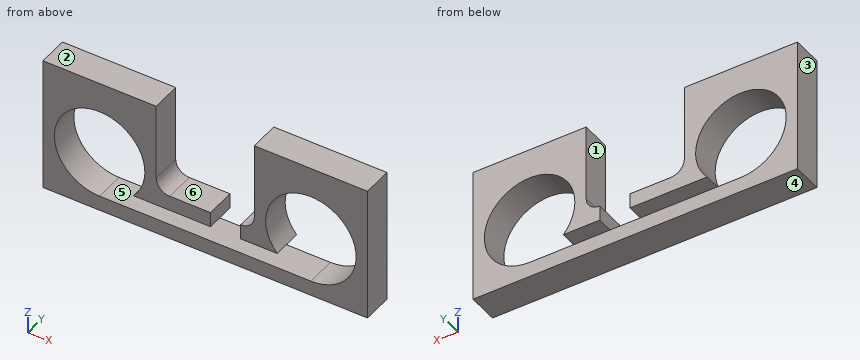
```python
from build123d import *

# Parameters (mm, degrees)
F0_W     = 273.05
F0_H     = 114.3
F1_DEPTH = 25.4
F2_R     = 38.1
F3_DEPTH = 25.4
F5_DEPTH = 25.4
F7_DEPTH = 25.4


with BuildPart() as f1:
    # F0 (on Front) → F1 (new body)
    with BuildSketch(Plane.XZ):
        with Locations((136.525, 57.15)):
            Rectangle(F0_W, F0_H)
    extrude(amount=F1_DEPTH)

    # F2 (on face) → F3 (cut)
    with BuildSketch(Plane.XZ.offset(25.4)):
        with Locations((47.625, 50.8)):
            Circle(F2_R)
        with Locations((225.425, 50.8)):
            Circle(F2_R)
    extrude(amount=-F3_DEPTH, mode=Mode.SUBTRACT)

    # F4 (on face) → F5 (cut)
    with BuildSketch(Plane.XZ.offset(25.4)):
        with BuildLine():
            Line((177.8, 114.3), (95.25, 114.3))
            Line((95.25, 114.3), (95.25, 49.53))
            ThreePointArc((95.25, 49.53), (98.597769, 41.447769), (106.68, 38.1))
            Line((106.68, 38.1), (166.37, 38.1))
            ThreePointArc((166.37, 38.1), (174.452231, 41.447769), (177.8, 49.53))
            Line((177.8, 49.53), (177.8, 114.3))
        make_face()
    extrude(amount=-F5_DEPTH, mode=Mode.SUBTRACT)

    # F6 (on face) → F7 (cut)
    with BuildSketch(Plane.XZ.offset(25.4)):
        Polygon((166.37, 25.4), (166.37, 38.1), (140.97, 38.1), (140.97, 25.4), (76.023063, 25.4), (47.625, 12.7), (166.37, 12.7), align=None)
        Polygon((197.026937, 25.4), (166.37, 25.4), (166.37, 12.7), (225.425, 12.7), align=None)
    extrude(amount=-F7_DEPTH, mode=Mode.SUBTRACT)


solid = f1.part
```
Can you work these out from the model? Positions are in its coordinate system, mm. Face numbers are marked on the shaded views. A direction names the side the tool comes from. Give positions to 0.01 mm unless a question says otherwise; leave off trailing zeros. Order: outer loops, then holes, each group sorted by start corner. A loop starts at its lowest first (then second) coordinate and runs counter-clockwise, first axis right, second up. Notation, with made-up numbers: (77.5, -18) - (130.5, -18) arc R17 cw to (130.5, -3) - close; hole circle Ø2 at (47.5, 7.5). An arc over 180 degrees is marked (long way). Use a Markdown table: item, result. Add a question column.
Q1. If we section it at A-A on z = 106: Write out the boundary of the cut face in (x, y).
Q2. If we mould it in two halves opening along X, with no side actions, what happens to the marked faces 1, 2 and 3? For each: released by +X, released by -X, zero draft, split by the parting line, or undercut.
Q3. If we section it at B-B on x = 243.5: Write out the boundary of the cut face in (y, z).
Q4. If we section it at D-D on y = -19: Write out the boundary of the cut face in (x, z) (3 decimals).
Q5. I'm going to push flat-ended pins straight in: pin 1 (12.5 mm diameter, centred on y = -6.5, z = 94, fed in from -X); pin 2 (7.5 mm diameter, centred on x = 124, y = -12.5, fed in from +Z); pin 3 (2 mm diameter, centred on x = 157, y = -17, fed in from +Z); pin 4 (2 mm diameter, centred on x = 244, z = 20.5, fed in from +Y). Where does each tip first touch, or does it pass through?
Q6. On a 3-axis mill with a long thin cutter (end or side, diameter ignored), from which of +Z, -Z, +X, -X, +Y, -Y can I reach the whole of each face in a straight line? I mean the marked faces 4, 5 and 6. Say none if no direction works.
Q7. If we section it at C-C on z = 58.5: Write out the boundary of the cut face in (x, y), plus the area to 3 significant figures.
Q8. Please list where these lines run through material, in increasing order: line 1 along X through (y, z) = (-11.75, 50.8) (3 decimals); line 2 along X through (y, z) = (-24.5, 100); line 3 along X through (y, z) = (-15.25, 86).
Answers follow:
| question | item | result |
|---|---|---|
| 1 | outline | (0, -25.4) - (95.25, -25.4) - (95.25, 0) - (0, 0) - close; (177.8, -25.4) - (273.05, -25.4) - (273.05, 0) - (177.8, 0) - close |
| 2 | face 1 | undercut |
| 2 | face 2 | zero draft |
| 2 | face 3 | released by -X |
| 3 | outline | (-25.4, 0) - (0, 0) - (0, 17.26) - (-25.4, 17.26) - close; (-25.4, 84.34) - (0, 84.34) - (0, 114.3) - (-25.4, 114.3) - close |
| 4 | outline | (0, 0) - (273.05, 0) - (273.05, 114.3) - (177.8, 114.3) - (177.8, 49.53) arc R11.43 cw to (166.37, 38.1) - (166.37, 25.4) - (197.027, 25.4) arc R38.1 cw (long way) to (225.425, 12.7) - (47.625, 12.7) arc R38.1 cw (long way) to (76.023, 25.4) - (140.97, 25.4) - (140.97, 38.1) - (106.68, 38.1) arc R11.43 cw to (95.25, 49.53) - (95.25, 114.3) - (0, 114.3) - close |
| 5 | pin 1 | stops at x = 0 |
| 5 | pin 2 | stops at z = 38.1 |
| 5 | pin 3 | stops at z = 12.7 |
| 5 | pin 4 | passes through |
| 6 | face 4 | -Z, +X, -X, +Y, -Y |
| 6 | face 5 | +Y, -Y |
| 6 | face 6 | +Z, +Y, -Y |
| 7 | outline | (0, -25.4) - (10.31, -25.4) - (10.31, 0) - (0, 0) - close; (84.94, -25.4) - (95.25, -25.4) - (95.25, 0) - (84.94, 0) - close; (177.8, -25.4) - (188.11, -25.4) - (188.11, 0) - (177.8, 0) - close; (262.74, -25.4) - (273.05, -25.4) - (273.05, 0) - (262.74, 0) - close |
| 7 | area | 1,050 mm^2 |
| 8 | line 1 | x = 0 to 9.525, 85.725 to 95.25, 177.8 to 187.325, 263.525 to 273.05 |
| 8 | line 2 | x = 0 to 95.25, 177.8 to 273.05 |
| 8 | line 3 | x = 0 to 33.05, 62.2 to 95.25, 177.8 to 210.85, 240 to 273.05 |
